Drawing for the job (mm, zero at the part's lowest x, y, z). A direction names the side the tool comes from. Give positions to 0.01 mm unless a question says otherwise; leave off trailing zeros. Loops run counter-clockwise (first coordinate to the right, second up) from the corner with the lowest first, then second, coordinate; pieces in that order, holes last. Notation, with made-up numbers: (-37, -18) -> (-20, -18) arc R14 cw to (-20, -9) -> close; hole circle Ø2 at (32.5, 88). An arc over 180 degrees is marked (long way). Answer in a Markdown table with one row per item. Add a question column.
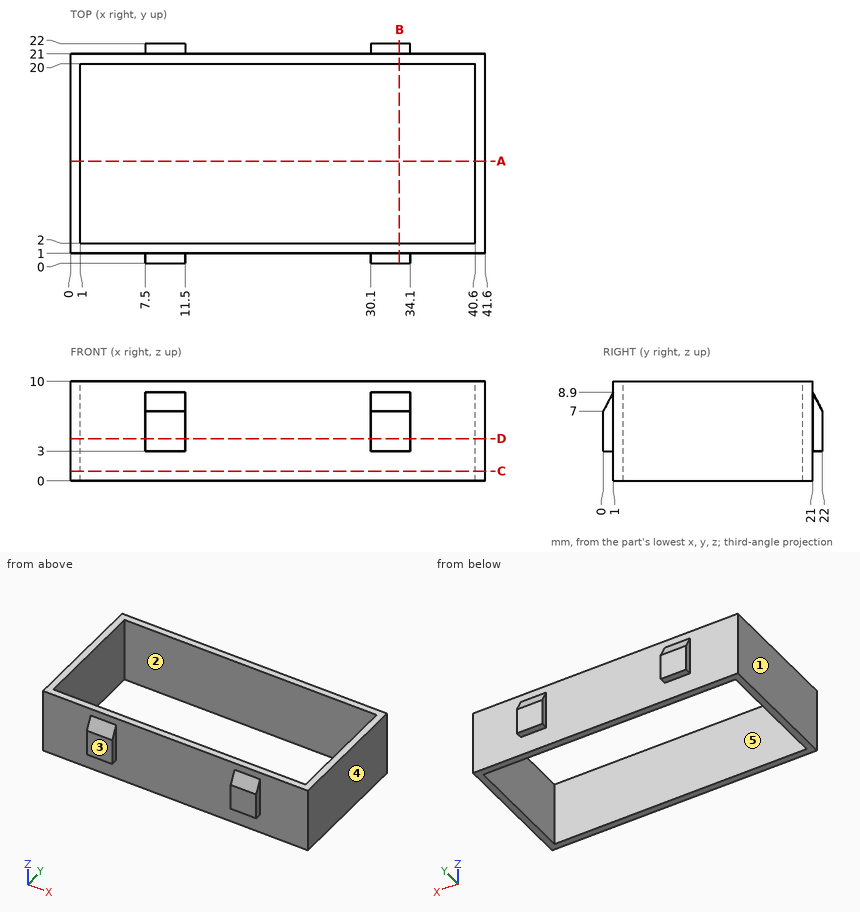
(1) Saw through at D-D, the plane z = 4.25. List the corners of the cut face in (x, y).
(2) Two-plate mould, pull along Y, no slides. Class the marked faces 1, 2 and 3: released by +Y, released by -Y, zero draft, split by the parting line, or undercut.
(3) Saw through at A-A, the plane y = 10.25. List the corners of the cut face in (x, z), then the cut area to 3 significant figures.
(4) Wall check: line 1 along Y through (x, z) = (33.5, 6.5); line 2 along Y through (x, z) = (12.5, 2.75); line 3 along X through (y, z) = (11, 3.75). Give the ranges that are in metal, low to high. Write a range as from..to.
(5) Flat gauge pins, fed straight in: pin 1 Ø0.5 at (y, z) = (21.5, 6.5) entering from -X; pin 2 Ø0.8 at (x, y) = (9.5, 21.5) entering from -Z; pin 3 Ø4 at (y, z) = (8, 4.5) entering from -X; pin 4 Ø5 at (x, z) = (25.5, 3) entering from -Y. Where does each tip first touch, or does it go through?
(6) Saw through at B-B, the plane x = 33. List the corners of the cut face in (y, z).
(7) Saw through at C-C, the plane z = 1. List the corners of the cut face in (x, y).
(8) 3-axis set-ups, long thin cutter, end or side, ignore diameter. For the marked faces 4 and 5: which of +Z, -Z, +X, -X, +Y, -Y reach the whole face in a straight line?
Worked answers:
| question | item | result |
|---|---|---|
| 1 | outline | (0, 1) -> (7.5, 1) -> (7.5, 0) -> (11.5, 0) -> (11.5, 1) -> (30.1, 1) -> (30.1, 0) -> (34.1, 0) -> (34.1, 1) -> (41.6, 1) -> (41.6, 21) -> (34.1, 21) -> (34.1, 22) -> (30.1, 22) -> (30.1, 21) -> (11.5, 21) -> (11.5, 22) -> (7.5, 22) -> (7.5, 21) -> (0, 21) -> close; hole (1, 2) -> (40.6, 2) -> (40.6, 20) -> (1, 20) -> close |
| 2 | face 1 | zero draft |
| 2 | face 2 | undercut |
| 2 | face 3 | released by -Y |
| 3 | outline | (0, 0) -> (1, 0) -> (1, 10) -> (0, 10) -> close; (40.6, 0) -> (41.6, 0) -> (41.6, 10) -> (40.6, 10) -> close |
| 3 | area | 20.0 mm^2 |
| 4 | line 1 | 0..2, 20..22 |
| 4 | line 2 | 1..2, 20..21 |
| 4 | line 3 | 0..1, 40.6..41.6 |
| 5 | pin 1 | x = 7.5 |
| 5 | pin 2 | z = 3 |
| 5 | pin 3 | x = 0 |
| 5 | pin 4 | y = 1 |
| 6 | outline | (0, 3) -> (1, 3) -> (1, 0) -> (2, 0) -> (2, 10) -> (1, 10) -> (1, 8.9) -> (0, 7) -> close; (20, 0) -> (21, 0) -> (21, 3) -> (22, 3) -> (22, 7) -> (21, 8.9) -> (21, 10) -> (20, 10) -> close |
| 7 | outline | (0, 1) -> (41.6, 1) -> (41.6, 21) -> (0, 21) -> close; hole (1, 2) -> (40.6, 2) -> (40.6, 20) -> (1, 20) -> close |
| 8 | face 4 | +Z, -Z, +X, +Y, -Y |
| 8 | face 5 | +Z, -Z |
